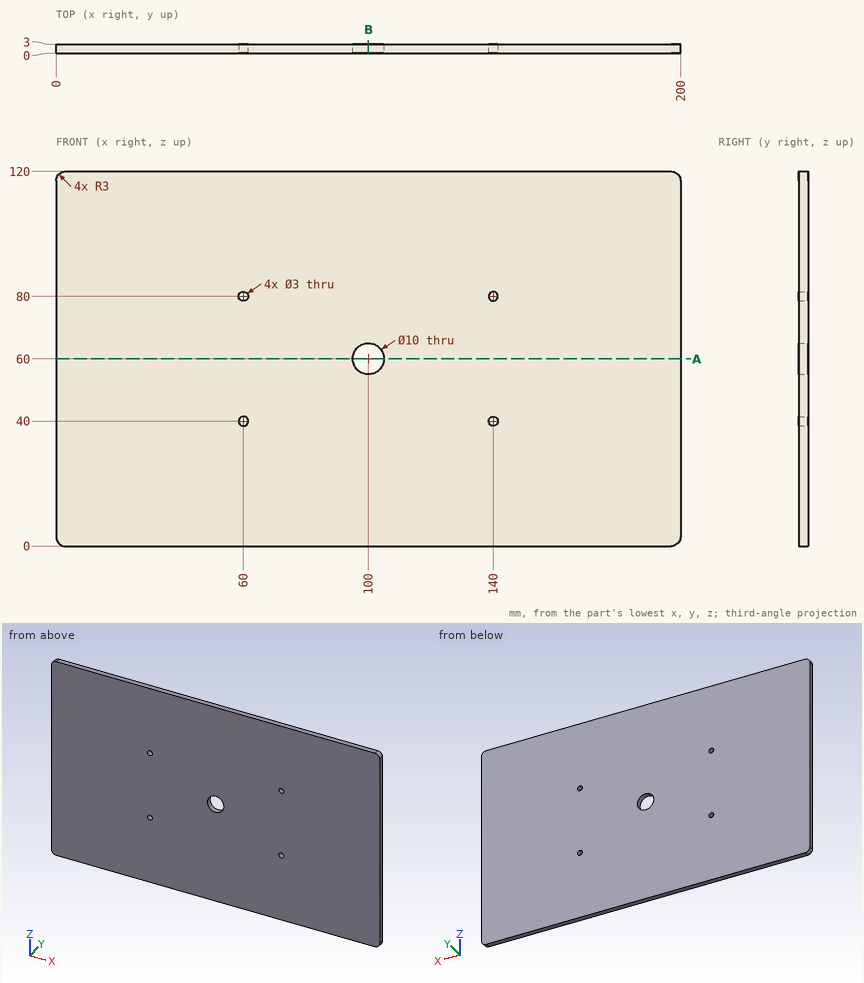
Here's the drawing with two shaded views (mm, measured from the low corner). I have some questions. Round coordinates to 2 decimals unless told otherwise and drop trailing zeros. Loops run counter-clockwise (first coordinate to the right, second up) from the corner with the lowest first, then second, coordinate; pieces in that order, holes last.
1. Suppose I cut it at A-A, the plane z = 60. Please give me the cut outline in (x, y).
Answers:
outline: (0, 0) - (95, 0) - (95, 3) - (0, 3) - close; (105, 0) - (200, 0) - (200, 3) - (105, 3) - close
2. Suppose I cut it at B-B, the plane x = 100. Please give me the cut outline in (y, z), and give its area (3 significant figures).
Answers:
outline: (0, 0) - (3, 0) - (3, 55) - (0, 55) - close; (0, 65) - (3, 65) - (3, 120) - (0, 120) - close
area: 330 mm2
3. If I drill on probe 1 along Z at (x, y) = (60, 0.95); probe 2 along X at (y, z) = (1, 80); probe 3 along Z at (x, y) = (100, 0.9), over which ranges is the centre line in solid material (lowest first)?
Answers:
probe 1: z = 0 to 38.5, 41.5 to 78.5, 81.5 to 120
probe 2: x = 0 to 58.5, 61.5 to 138.5, 141.5 to 200
probe 3: z = 0 to 55, 65 to 120
4. Will this pin go through, and if not, where does the flat tip stop? pin 1 (4 mm diameter, centred on x = 140, z = 80, fed in from -Y).
Answers:
pin 1: stops at y = 0
